from build123d import *

# Parameters (mm, degrees)
SKETCH_AS_DRAWN_W              = 30
SKETCH_AS_DRAWN_H              = 15
SKETCH_AS_DRAWN_R              = 2.7
EXTRUDE_DEPTH                  = 10
EXTRUDE_ONTO_SKETCH_ROLL_ANGLE = 90
SKETCH001_R                    = 2.7
POCKET_DEPTH                   = 15.001
SKETCH002_W                    = 8.2
SKETCH002_H                    = 4.5
POCKET001_DEPTH                = 10.001
SKETCH003_W                    = 10
SKETCH003_H                    = 10
PAD_DEPTH                      = 12
SKETCH004_R                    = 2.7
POCKET002_DEPTH                = 27.001


with BuildPart() as part:
    # Sketch as drawn → Extrude (new)
    with BuildSketch(Plane.XY):
        with Locations((15, 7.5)):
            Rectangle(SKETCH_AS_DRAWN_W, SKETCH_AS_DRAWN_H)
        with Locations((5, 5)):
            Circle(SKETCH_AS_DRAWN_R, mode=Mode.SUBTRACT)
        with Locations((25, 5)):
            Circle(SKETCH_AS_DRAWN_R, mode=Mode.SUBTRACT)
    extrude(amount=-EXTRUDE_DEPTH)


with BuildPart() as part_1:
    # Extrude onto Sketch roll: moved
    add(part.part.rotate(Axis((0, 0, 0), (1, 0, 0)), EXTRUDE_ONTO_SKETCH_ROLL_ANGLE))


with BuildPart() as part_2:
    # Extrude onto Sketch placement: moved
    add(part_1.part)

    # Sketch001 → Pocket (cut, through all)
    with BuildSketch(Plane.XY.offset(15)):
        with Locations((15, 5)):
            Circle(SKETCH001_R)
    extrude(amount=-POCKET_DEPTH, mode=Mode.SUBTRACT)

    # Sketch002 → Pocket001 (cut, through all)
    with BuildSketch(Plane.XZ):
        with Locations((14.263317, 7.25)):
            Rectangle(SKETCH002_W, SKETCH002_H)
    extrude(amount=-POCKET001_DEPTH, mode=Mode.SUBTRACT)

    # Sketch003 → Pad (new body)
    with BuildSketch(Plane(origin=(0, 0, 0), x_dir=(1, 0, 0), z_dir=(0, 0, -1))):
        with Locations((15, -5)):
            Rectangle(SKETCH003_W, SKETCH003_H)
    extrude(amount=PAD_DEPTH)

    # Sketch004 → Pocket002 (cut, through all)
    with BuildSketch(Plane(origin=(0, 0, -12), x_dir=(1, 0, 0), z_dir=(0, 0, -1))):
        with Locations((15, -5)):
            Circle(SKETCH004_R)
    extrude(amount=-POCKET002_DEPTH, mode=Mode.SUBTRACT)


solid = part_2.part
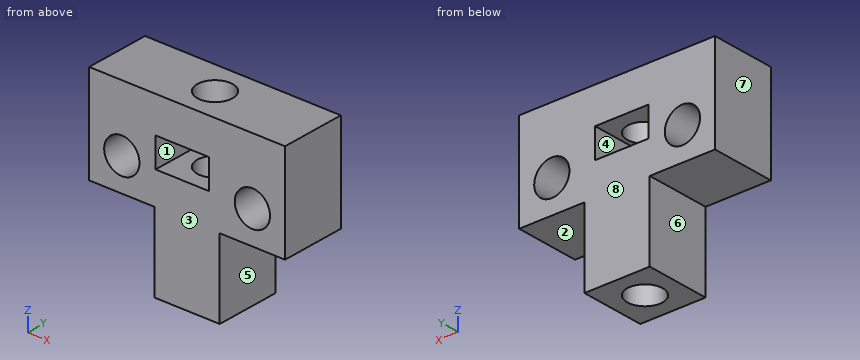
The model under review builds one solid part; all positions refer to its coordinate system, in mm. Face numbers are marked on the shaded views. A direction names the side the tool comes from. Round coordinates to 2 decimals unless told otherwise and drop trailing zeros. Loops run counter-clockwise (first coordinate to the right, second up) from the corner with the lowest first, then second, coordinate; pieces in that order, holes last. Notation, with made-up numbers: (87.25, -37) -> (110.25, -37) arc R12 cw to (110.25, -29) -> close; hole circle Ø10 at (25, 65). An arc over 180 degrees is marked (long way). Write item = value, one per line. Start each with the question number.
Item 1: To check wall thickness, follow L1, parallel to Y at x = 15, z = -7; L2, parallel to Z at x = 25, y = 7; L3, parallel to X at y = 6.5, z = 5.75. State the ranges of each line that lie inside material, in increasing order.
Item 2: Take a section at D-D on y = 8.75. Give the boundary of the cut face in (x, z), plus the area to 3 significant figures.
Item 3: Take a section at B-B on y = 5. Give the boundary of the cut face in (x, z).
Item 4: Insertion check: pin 1 (5 mm diameter, centred on y = 4.5, z = -6, fed in from +X); pin 2 (3 mm diameter, centred on y = 6, z = -8, fed in from -X); pin 3 (5 mm diameter, centred on x = 5.5, y = 3, fed in from -Z). Each pin has a flat end and moves straight along its axis. Give the tip position at first contact, or say it passes through.
Item 5: Mouldability with a two-part tool opening along Z and no side actions: class the marked faces 1, 2 and 3 as released by +Z, released by -Z, zero draft, split by the parting line, or undercut.
Item 6: Take a section at C-C on z = 9. Give the boundary of the cut face in (x, y).
Item 7: For the marked faces 4, 5, 6, 7 and 8, list the 3-axis set-ups (+Z, -Z, +X, -X, +Y, -Y) from which the entire face can be reached by the end or side of a thin tool; tool diameter is ignored.
Item 8: Take a section at A-A on x = 5. Give the boundary of the cut face in (y, z), plus the area to 3 significant figures.
Result:
q1.L1 = 0 to 2.3, 7.7 to 10
q1.L2 = 0 to 2.3, 7.7 to 15
q1.L3 = 0 to 2.41, 7.59 to 10.16, 18.36 to 22.41, 27.59 to 30
q2.outline = (0, 0) -> (10, 0) -> (10, -12) -> (20, -12) -> (20, 0) -> (30, 0) -> (30, 15) -> (0, 15) -> close; hole circle Ø5.4 at (5, 5); hole (10.16, 5) -> (18.36, 5) -> (18.36, 9.5) -> (10.16, 9.5) -> close; hole circle Ø5.4 at (25, 5)
q2.area = 487 mm²
q3.outline = (0, 0) -> (10, 0) -> (10, -12) -> (12.3, -12) -> (12.3, 5) -> (10.16, 5) -> (10.16, 9.5) -> (12.3, 9.5) -> (12.3, 15) -> (0, 15) -> close; (17.7, -12) -> (20, -12) -> (20, 0) -> (30, 0) -> (30, 15) -> (17.7, 15) -> (17.7, 9.5) -> (18.36, 9.5) -> (18.36, 5) -> (17.7, 5) -> close; hole circle Ø5.4 at (5, 5); hole circle Ø5.4 at (25, 5)
q4.pin_1 = 20
q4.pin_2 = 10
q4.pin_3 = 0
q5.face_1 = undercut
q5.face_2 = released by -Z
q5.face_3 = zero draft
q6.outline = (0, 0) -> (10.16, 0) -> (10.16, 10) -> (0, 10) -> close; (18.36, 0) -> (30, 0) -> (30, 10) -> (18.36, 10) -> close
q7.face_4 = +Y, -Y
q7.face_5 = -Z, +X, +Y, -Y
q7.face_6 = -Z, -X, +Y, -Y
q7.face_7 = +Z, -Z, -X, +Y, -Y
q7.face_8 = +Z, -Z, +X, -X, +Y
q8.outline = (0, 0) -> (10, 0) -> (10, 2.3) -> (0, 2.3) -> close; (0, 7.7) -> (10, 7.7) -> (10, 15) -> (0, 15) -> close
q8.area = 96.0 mm²
